```python
from build123d import *

# Parameters (mm, degrees)
F0_R     = 5
F1_DEPTH = 3
F2_D     = 3


with BuildPart() as f1:
    # F0 (on Front) → F1 (new body)
    with BuildSketch(Plane.XZ):
        with BuildLine():
            Line((29.2013126835, 21), (-40.7986873165, 21))
            Line((-40.7986873165, 21), (-40.7986873165, 12))
            Line((-40.7986873165, 12), (-10.7986873165, 12))
            ThreePointArc((-10.7986873165, 12), (-7.2631534106, 10.5355339059), (-5.7986873165, 7))
            Line((-5.7986873165, 7), (-5.7986873165, -7))
            ThreePointArc((-5.7986873165, -7), (-7.2631534106, -10.5355339059), (-10.7986873165, -12))
            Line((-10.7986873165, -12), (-40.7986873165, -12))
            Line((-40.7986873165, -12), (-40.7986873165, -21))
            Line((-40.7986873165, -21), (29.2013126835, -21))
            Line((29.2013126835, -21), (29.2013126835, -4.5))
            ThreePointArc((29.2013126835, -4.5), (15.7013126835, 0), (29.2013126835, 4.5))
            Line((29.2013126835, 4.5), (29.2013126835, 21))
        make_face()
        with BuildLine():
            Line((-2.2986873165, -17.05), (-36.2986873165, -17.05))
            ThreePointArc((-36.2986873165, -17.05), (-37.8486873165, -15.5), (-36.2986873165, -13.95))
            Line((-36.2986873165, -13.95), (-2.2986873165, -13.95))
            ThreePointArc((-2.2986873165, -13.95), (-1.2026718057, -14.4039844892), (-0.7486873165, -15.5))
            ThreePointArc((-0.7486873165, -15.5), (-1.2026718057, -16.5960155108), (-2.2986873165, -17.05))
        make_face(mode=Mode.SUBTRACT)
        with BuildLine():
            ThreePointArc((-36.2986873165, 13.95), (-37.8486873165, 15.5), (-36.2986873165, 17.05))
            Line((-36.2986873165, 17.05), (-2.2986873165, 17.05))
            ThreePointArc((-2.2986873165, 17.05), (-1.2026718057, 16.5960155108), (-0.7486873165, 15.5))
            ThreePointArc((-0.7486873165, 15.5), (-1.2026718057, 14.4039844892), (-2.2986873165, 13.95))
            Line((-2.2986873165, 13.95), (-36.2986873165, 13.95))
        make_face(mode=Mode.SUBTRACT)
        with BuildLine():
            ThreePointArc((30.7013126835, 0), (30.3164374189, 2.3717082451), (29.2013126835, 4.5))
            Line((29.2013126835, 4.5), (29.2013126835, -4.5))
            ThreePointArc((29.2013126835, -4.5), (30.3164374189, -2.3717082451), (30.7013126835, 0))
        make_face()
        with BuildLine():
            Line((29.2013126835, -4.5), (29.2013126835, 4.5))
            ThreePointArc((29.2013126835, 4.5), (15.7013126835, 0), (29.2013126835, -4.5))
        make_face()
        with Locations((23.2013126835, 0)):
            Circle(F0_R, mode=Mode.SUBTRACT)
    extrude(amount=F1_DEPTH)

    # F2 (through all)
    with Locations(Plane(origin=(0, 0, 0), x_dir=(1, 0, 0), z_dir=(0, 1, 0))):
        with Locations((16.2013126835, 18.875), (26.2013126835, 18.875)):
            Hole(F2_D / 2)


solid = f1.part
```
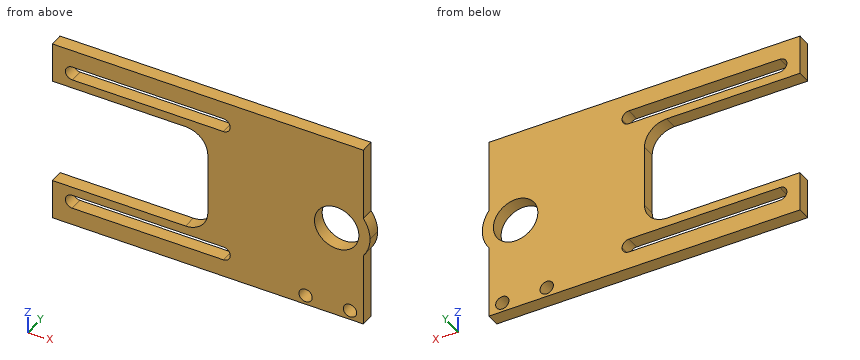
The listing builds one solid part. Answer for the finished solid, in the listing's coordinates (mm). Give positions to 0.01 mm unless a question says otherwise; leave off trailing zeros. Order: outer loops, then holes, each group sorted by start corner. A loop starts at its lowest first (then second) coordinate and runs counter-clockwise, first axis right, second up.
Item 1: The part is cut by section B-B, the plane z = 2. Give the vertices of the cut face in (x, y), and give its area (3 significant figures).
From the geometry:
outline: (-5.8, -3) - (18.62, -3) - (18.62, 0) - (-5.8, 0) - close; (27.78, -3) - (30.43, -3) - (30.43, 0) - (27.78, 0) - close
area: 81.2 mm2
Item 2: The part is cut by section A-A, the plane x = -23. Give the vertices of the cut face in (y, z).
From the geometry:
outline: (-3, -21) - (0, -21) - (0, -17.05) - (-3, -17.05) - close; (-3, -13.95) - (0, -13.95) - (0, -12) - (-3, -12) - close; (-3, 12) - (0, 12) - (0, 13.95) - (-3, 13.95) - close; (-3, 17.05) - (0, 17.05) - (0, 21) - (-3, 21) - close
Item 3: Given pin 1 Ø6 at (x, z) = (23.2, 0) entering from +Y; pin 2 Ø1.5 at (y, z) = (-1, -3) entering from -X, each flat-ended and moving along its own axis, determine where each tip first touches the part or whether it passes through.
From the geometry:
pin 1: passes through
pin 2: stops at x = -5.8
Item 4: The part is cut by section D-D, the plane y = -1.7. Give the vertices of the cut face in (x, z) (3 decimals), and give its area (3 significant figures).
From the geometry:
outline: (-40.799, -21) - (29.201, -21) - (29.201, -4.5) arc R7.5 ccw to (29.201, 4.5) - (29.201, 21) - (-40.799, 21) - (-40.799, 12) - (-10.799, 12) arc R5 cw to (-5.799, 7) - (-5.799, -7) arc R5 cw to (-10.799, -12) - (-40.799, -12) - close; hole (-36.299, -17.05) - (-2.299, -17.05) arc R1.55 ccw to (-2.299, -13.95) - (-36.299, -13.95) arc R1.55 ccw to start; hole (-36.299, 13.95) - (-2.299, 13.95) arc R1.55 ccw to (-2.299, 17.05) - (-36.299, 17.05) arc R1.55 ccw to start; hole circle Ø3 at (16.201, -18.875); hole circle Ø10 at (23.201, 0); hole circle Ø3 at (26.201, -18.875)
area: 1,800 mm2
Item 5: Find the intervals of material crossed by probe 1 along Z at (x, y) = (-15.5, -0.95); probe 2 along Z at (x, y) = (-3, -0.7); probe 3 along X at (y, z) = (-2.7, -15.5), in increasing order.
From the geometry:
probe 1: z = -21 to -17.05, -13.95 to -12, 12 to 13.95, 17.05 to 21
probe 2: z = -21 to -17.05, -13.95 to 13.95, 17.05 to 21
probe 3: x = -40.8 to -37.85, -0.75 to 29.2
Item 6: The part is cut by section C-C, the plane x = -4. Give the vertices of the cut face in (y, z), and give its area (3 significant figures).
From the geometry:
outline: (-3, -21) - (0, -21) - (0, -17.05) - (-3, -17.05) - close; (-3, -13.95) - (0, -13.95) - (0, 13.95) - (-3, 13.95) - close; (-3, 17.05) - (0, 17.05) - (0, 21) - (-3, 21) - close
area: 107 mm2
